Read the model definition and answer for the solid it produces. Units are mm, in the model's axes. A direction names the side the tool comes from. Coordinates: 2 decimals unless noted, no trailing zeros. Loops run counter-clockwise (first coordinate to the right, second up) from the corner with the lowest first, then second, coordinate; pieces in that order, holes last.
from build123d import *

# Parameters (mm, degrees)
SKETCH1_W               = 44.45
SKETCH1_H               = 120.65
BOSS_EXTRUDE1_DEPTH     = 190.5
SKETCH2_W               = 38.1
SKETCH2_H               = 107.95
CUT_EXTRUDE1_DEPTH      = 184.15
CUT_EXTRUDE4_DEPTH      = 199.811796997
CUT_EXTRUDE4_DEPTH_BACK = 199.811796997
SKETCH4_R               = 3.2385
SKETCH17_W              = 6.477
SKETCH17_H              = 38.227
CUT_EXTRUDE5_DEPTH      = 230.8314056
SKETCH18_W              = 50.8
SKETCH18_H              = 50.8
CUT_EXTRUDE6_DEPTH      = 204.423119691
SKETCH19_W              = 44.45
SKETCH19_H              = 6.35
BOSS_EXTRUDE2_DEPTH     = 12.7
SKETCH21_R              = 2.063500064
SKETCH21_R_2            = 2.063499937
CUT_EXTRUDE7_DEPTH      = 204.02629294
SKETCH23_R              = 4.063500001
CUT_EXTRUDE8_DEPTH      = 209.803024703
SKETCH24_R              = 1.000000032
CUT_EXTRUDE9_DEPTH      = 237.745168905
SKETCH25_R              = 1.000000032
CUT_EXTRUDE10_DEPTH     = 237.745168905
LPATTERN1_COUNT         = 2
LPATTERN1_PITCH         = 57.15


with BuildPart() as part:
    # Sketch1 → Boss-Extrude1 (new body)
    with BuildSketch(Plane.XY):
        with Locations((22.225, 0)):
            Rectangle(SKETCH1_W, SKETCH1_H)
    extrude(amount=BOSS_EXTRUDE1_DEPTH)

    # Sketch2 → Cut-Extrude1 (cut)
    with BuildSketch(Plane(origin=(0, 0, 0), x_dir=(-1, 0, 0), z_dir=(0, 0, -1))):
        with Locations((-25.4, 0)):
            Rectangle(SKETCH2_W, SKETCH2_H)
    extrude(amount=-CUT_EXTRUDE1_DEPTH, mode=Mode.SUBTRACT)

    # Sketch4 → Cut-Extrude4 (cut, two sides: drawn at the far end of the back side and taken through both)
    with BuildSketch(Plane(origin=(0, 0, 184.15), x_dir=(-1, 0, 0), z_dir=(0, 0, -1)).offset(-CUT_EXTRUDE4_DEPTH_BACK)):
        with Locations((-38.1, 38.1)):
            Circle(SKETCH4_R)
        with Locations(Location((-38.1, -38.1, 0), (0, 0, 180))):
            Circle(SKETCH4_R)
    extrude(amount=CUT_EXTRUDE4_DEPTH + CUT_EXTRUDE4_DEPTH_BACK, mode=Mode.SUBTRACT)

    # Sketch17 → Cut-Extrude5 (cut, through all)
    with BuildSketch(Plane.XZ.offset(60.325)):
        with Locations((41.2115, 133.2865)):
            Rectangle(SKETCH17_W, SKETCH17_H)
    extrude(amount=-CUT_EXTRUDE5_DEPTH, mode=Mode.SUBTRACT)

    # Sketch18 → Cut-Extrude6 (cut, through all)
    with BuildSketch(Plane(origin=(6.35, 0, 0), x_dir=(0, 0, -1), z_dir=(1, 0, 0))):
        with Locations((-25.4, 0)):
            Rectangle(SKETCH18_W, SKETCH18_H)
    extrude(amount=-CUT_EXTRUDE6_DEPTH, mode=Mode.SUBTRACT)

    # Sketch19 → Boss-Extrude2 (add)
    with BuildSketch(Plane.XZ.offset(60.325)):
        with Locations((22.225, 3.175)):
            Rectangle(SKETCH19_W, SKETCH19_H)
    boss_extrude2 = extrude(amount=BOSS_EXTRUDE2_DEPTH)

    # Sketch21 → Cut-Extrude7 (cut, through all)
    with BuildSketch(Plane.XY.offset(6.35)):
        with Locations((6.35, -67.197573915)):
            Circle(SKETCH21_R)
        with Locations((38.1, -67.197573915)):
            Circle(SKETCH21_R_2)
    cut_extrude7 = extrude(amount=-CUT_EXTRUDE7_DEPTH, mode=Mode.SUBTRACT)

    # Mirror1: Boss-Extrude2, Cut-Extrude7 across plane
    add(boss_extrude2.mirror(Plane.ZX))
    add(cut_extrude7.mirror(Plane.ZX), mode=Mode.SUBTRACT)

    # Sketch23 → Cut-Extrude8 (cut, through all)
    with BuildSketch(Plane.XY.offset(190.5)):
        with Locations((20.7499966, 0)):
            Circle(SKETCH23_R)
    extrude(amount=-CUT_EXTRUDE8_DEPTH, mode=Mode.SUBTRACT)

    # Sketch24 → Cut-Extrude9 (cut, through all)
    with BuildSketch(Plane.XZ.offset(60.325)):
        with Locations(Location((12.7, 117.348, 0), (0, 0, 270))):
            Circle(SKETCH24_R)
        with Locations(Location((12.7, 136.398, 0), (0, 0, 270))):
            Circle(SKETCH24_R)
    extrude(amount=-CUT_EXTRUDE9_DEPTH, mode=Mode.SUBTRACT)

    # Sketch25 → Cut-Extrude10 (cut, through all)
    with BuildSketch(Plane.XZ.offset(60.325)):
        with Locations(Location((9.525, 156.21, 0), (0, 0, 270))):
            Circle(SKETCH25_R)
        with Locations(Location((34.925, 156.21, 0), (0, 0, 270))):
            Circle(SKETCH25_R)
        with Locations(Location((34.925, 165.1, 0), (0, 0, 270))):
            Circle(SKETCH25_R)
        with Locations(Location((9.525, 165.1, 0), (0, 0, 270))):
            Circle(SKETCH25_R)
    cut_extrude10 = extrude(amount=-CUT_EXTRUDE10_DEPTH, mode=Mode.SUBTRACT)

    # LPattern1: Cut-Extrude10 ×2
    with Locations(*[(0, 0, -i * LPATTERN1_PITCH) for i in range(1, LPATTERN1_COUNT)]):
        add(cut_extrude10, mode=Mode.SUBTRACT)


solid = part.part
Q1. A cutting plane is placed at D-D (z = 175). Give the vertices of the cut face in (x, y) (3 decimals), then the cut area to 3 significant figures.
Findings below:
outline: (0, -60.325) - (44.45, -60.325) - (44.45, -53.975) - (6.35, -53.975) - (6.35, 53.975) - (44.45, 53.975) - (44.45, 60.325) - (0, 60.325) - close
area: 1,250 mm2
Q2. Which of the six approach directions +Z, -Z, +X, -X, +Y, -Y give full straight-line access (tool end or side, diameter ignored) to faces 4 (the face through (26, 53.975, 91)), 5 (the face through (37.973, 57, 133)), 6 (the face through (22, -67, 6.35)), 7 (the face through (3, -25.4, 26))?
Findings below:
face 4: -Z, +X
face 5: +X, +Y, -Y
face 6: +Z, +X, -X, -Y
face 7: -Z, +X, -X
Q3. A cutting plane is placed at B-B (z = 46). Give the vertices of the cut face in (x, y) (3 decimals).
Findings below:
outline: (0, -60.325) - (44.45, -60.325) - (44.45, -53.975) - (6.35, -53.975) - (6.35, -25.4) - (0, -25.4) - close; (0, 25.4) - (6.35, 25.4) - (6.35, 53.975) - (44.45, 53.975) - (44.45, 60.325) - (0, 60.325) - close
Q4. A cutting plane is placed at C-C (x = 20). Give the vertices of the cut face in (y, z) (3 decimals).
Findings below:
outline: (-73.025, 0) - (-53.975, 0) - (-53.975, 184.15) - (-3.994, 184.15) - (-3.994, 190.5) - (-60.325, 190.5) - (-60.325, 6.35) - (-73.025, 6.35) - close; (3.994, 184.15) - (53.975, 184.15) - (53.975, 0) - (73.025, 0) - (73.025, 6.35) - (60.325, 6.35) - (60.325, 190.5) - (3.994, 190.5) - close
Q5. Flat-ended cylindrical pins translate along their axes: pin 1 Ø11.5 at (x, z) = (26, 89.5) entering from +Y (3 decimals); pin 2 Ø5 at (y, z) = (56.5, 131) entering from +X; pin 3 Ø5 at (x, y) = (9, 40.5) entering from -Z. Find the tip coordinate at first contact, or state that the pin passes through.
Findings below:
pin 1: stops at y = 60.325
pin 2: stops at x = 37.97
pin 3: stops at z = 184.15
Q6. Determine the mould class of faces 1 (the face through (36.5, -68.5, 3.2)), 2 (the face through (41, -57, 152.4)), 3 (the face through (0, -1, 94)) for opening direction X: +X half, -X half, draft (parallel to the pull), parting line (faces both ways), or undercut.
Findings below:
face 1: undercut
face 2: draft
face 3: -X half
Q7. A cutting plane is placed at A-A (y = 38.1). Give the vertices of the cut face in (x, z), then the cut area to 3 significant figures.
Findings below:
outline: (0, 0) - (6.35, 0) - (6.35, 184.15) - (34.86, 184.15) - (34.86, 190.5) - (0, 190.5) - close; (41.34, 184.15) - (44.45, 184.15) - (44.45, 190.5) - (41.34, 190.5) - close
area: 1,410 mm2
Q8. Straight lines are drawn through the part: probe 1 along X at (y, z) = (57.5, 156.21) (3 decimals); probe 2 along Y at (x, z) = (40.5, 43) (3 decimals); probe 3 along Z at (x, y) = (40.5, 58). For each, find the intervals that lie inside material, in ascending order.
Findings below:
probe 1: x = 0 to 8.525, 10.525 to 33.925, 35.925 to 44.45
probe 2: y = -60.325 to -53.975, 53.975 to 60.325
probe 3: z = 0 to 114.17, 152.4 to 190.5
